```python
from build123d import *

# Parameters (mm, degrees)
F0_R     = 6.74
F1_DEPTH = 38.4
F2_R     = 5.675
F3_DEPTH = 22.42
F4_R     = 5.625
F5_DEPTH = 12.5
F6_R     = 5.675
F7_DEPTH = 22.42
F8_R     = 5.625
F9_DEPTH = 12.5


with BuildPart() as f1:
    # F0 (on Front) → F1 (new body, symmetric)
    with BuildSketch(Plane.XZ):
        Circle(F0_R)
    extrude(amount=F1_DEPTH, both=True)

    # F2 (on face) → F3 (join)
    with BuildSketch(Plane(origin=(0, 38.4, 0), x_dir=(-1, 0, 0), z_dir=(0, 1, 0))):
        Circle(F2_R)
    extrude(amount=F3_DEPTH)

    # F4 (on face) → F5 (join)
    with BuildSketch(Plane(origin=(0, 60.82, 0), x_dir=(-1, 0, 0), z_dir=(0, 1, 0))):
        Circle(F4_R)
    extrude(amount=F5_DEPTH)

    # F6 (on face) → F7 (join)
    with BuildSketch(Plane.XZ.offset(38.4)):
        Circle(F6_R)
    extrude(amount=F7_DEPTH)

    # F8 (on face) → F9 (join)
    with BuildSketch(Plane.XZ.offset(60.82)):
        Circle(F8_R)
    extrude(amount=F9_DEPTH)


solid = f1.part
```
The model under review builds one solid part; all positions refer to its coordinate system, in mm. A direction names the side the tool comes from. Round coordinates to 2 decimals unless told otherwise and drop trailing zeros. Write each loop counter-clockwise with the first axis right and the second up, starting at its lowest first coordinate (ties: lowest second). Pieces come first, ordered by that corner, then holes.
(1) Machinability: for faces 1 (the cylindrical face through (6.226, -0.538, -2.581)), 2 (the cylindrical face through (-5.242, 49.453, -2.174)), 3 (the cylindrical face through (2.6, -66.98, -4.99)), which of the approach directions +Z, -Z, +X, -X, +Y, -Y give a long, thin tool a straight path to every point of the face, cutting with its end or side? Answer none if there is none.
(2) We need section C-C on y = -63.5. Give the boundary of the cut face in (x, z) (3 decimals), and give its area (3 significant figures).
(3) Mouldability with a two-part tool opening along Y and no side actions: class faces 4 (the flat face through (-3, 38.4, -5)), 5 (the flat face through (-3, -38.4, -5)), 6 (the cylindrical face through (5.242, -49.453, -2.174)) as +Y half, -Y half, draft (parallel to the pull), parting line (faces both ways), or undercut.
(4) We need section B-B on z = 0. Give the boundary of the cut face in (x, y) (3 decimals), and give its area (3 significant figures).
(5) Insertion check: pin 1 (6 mm diameter, centred on x = 4.5, y = 31.5, fed in from -Z); pin 2 (2 mm diameter, centred on x = -5, y = -2, fed in from -Z); pin 3 (1 mm diameter, centred on y = 34, z = -4.5, fed in from -X). Each pin has a flat end and moves straight along its axis. Give the tip position at first contact, or say it passes through.
(6) Wall thickness on L1, parallel to X at y = 20, z = 0.25; L2, parallel to X at y = -43, z = 0.75; L3, parallel to Y at x = -2.25, z = 6: over which ranges is each line inside the solid? List them lowest first.
(7) We need section D-D on y = 32.5. Give the boundary of the cut face in (x, z), and give its area (3 significant figures).
(8) We need section A-A on x = 0. Give the boundary of the cut face in (y, z) (3 decimals), and give its area (3 significant figures).
Findings below:
1. face 1: +Y, -Y
1. face 2: +Y
1. face 3: -Y
2. outline: circle Ø11.25 at (0, 0)
2. area: 99.4 mm2
3. face 4: +Y half
3. face 5: -Y half
3. face 6: draft
4. outline: (-6.74, -38.4) - (-5.675, -38.4) - (-5.675, -60.82) - (-5.625, -60.82) - (-5.625, -73.32) - (5.625, -73.32) - (5.625, -60.82) - (5.675, -60.82) - (5.675, -38.4) - (6.74, -38.4) - (6.74, 38.4) - (5.675, 38.4) - (5.675, 60.82) - (5.625, 60.82) - (5.625, 73.32) - (-5.625, 73.32) - (-5.625, 60.82) - (-5.675, 60.82) - (-5.675, 38.4) - (-6.74, 38.4) - close
4. area: 1,830 mm2
5. pin 1: stops at z = -6.57
5. pin 2: stops at z = -5.42
5. pin 3: stops at x = -5.42
6. L1: x = -6.74 to 6.74
6. L2: x = -5.63 to 5.63
6. L3: y = -38.4 to 38.4
7. outline: circle Ø13.48 at (0, 0)
7. area: 143 mm2
8. outline: (-73.32, -5.625) - (-60.82, -5.625) - (-60.82, -5.675) - (-38.4, -5.675) - (-38.4, -6.74) - (38.4, -6.74) - (38.4, -5.675) - (60.82, -5.675) - (60.82, -5.625) - (73.32, -5.625) - (73.32, 5.625) - (60.82, 5.625) - (60.82, 5.675) - (38.4, 5.675) - (38.4, 6.74) - (-38.4, 6.74) - (-38.4, 5.675) - (-60.82, 5.675) - (-60.82, 5.625) - (-73.32, 5.625) - close
8. area: 1,830 mm2
